Part model, mm, in its own coordinate system. Face numbers are marked on the shaded views. A direction names the side the tool comes from. Give positions to 0.01 mm unless a question says otherwise; leave off trailing zeros. Order: outer loops, then holes, each group sorted by start corner. A loop starts at its lowest first (then second) coordinate and runs counter-clockwise, first axis right, second up. Notation, with made-up numbers: M 11,29.5 L 34,29.5 A18 ccw 34,56.5 Z; hole C 4,79.5 d6. An arc over 180 degrees is marked long. One line per question, with ' | ' between items.
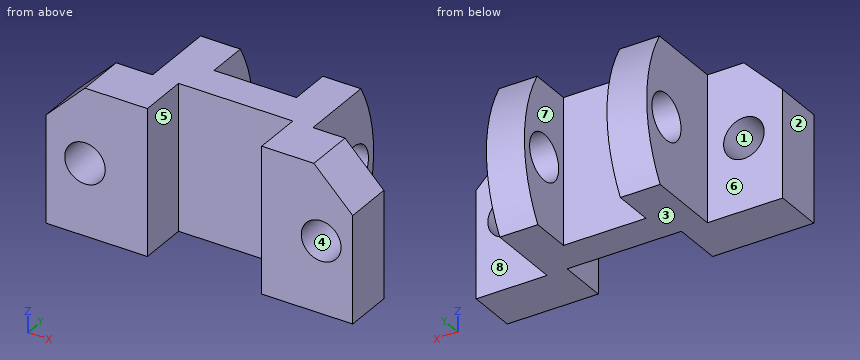
Autodesk Inventor part; units mm, degrees
ref_plane "YZ Plane" through (0, 0, 0) normal (1, 0, 0) x (0, 1, 0)
ref_plane "XZ Plane" through (0, 0, 0) normal (0, 1, 0) x (-1, 0, 0)
ref_plane "XY Plane" through (0, 0, 0) normal (0, 0, 1) x (1, 0, 0)
sketch "스케치1" plane through (0, 0, 0) normal (0, 0, 1) x (1, 0, 0)
  line L0 (31.5724, -15.0322) -> (-31.5724, -15.0322)
  line L1 (-31.5724, -15.0322) -> (-31.5724, 15.0322)
  line L2 (-31.5724, 15.0322) -> (31.5724, 15.0322)
  line L3 (31.5724, 15.0322) -> (31.5724, -15.0322)
  line L4 (31.5724, -15.0322) -> (-31.5724, 15.0322) construction
  line L5 (-31.5724, -15.0322) -> (31.5724, 15.0322) construction
  point P0 (0, 0)
extrude "돌출1" add sketch "스케치1" along normal blind 30
sketch "스케치2" plane through (-31.5724, 15.0322, 0) normal (0, 1, 0) x (1, 0, 0)
  point P0 (31.5724, 0)
sketch "스케치3" plane through (-31.5724, 15.0322, 0) normal (0, 1, 0) x (1, 0, 0)
  line L0 (63.1447, 0) -> (0, 0)
  line L1 (15.5145, 0) -> (15.5145, -30)
  line L2 (0, -30) -> (63.1447, -30)
  line L3 (48.5426, 0) -> (48.5426, -30)
  line L4 (63.1447, -30) -> (0, -30)
  line L5 (15.5145, -30) -> (0, -30)
  line L6 (0, 0) -> (63.1447, 0)
  line L7 (0, -30) -> (0, 0)
  line L8 (0, 0) -> (15.5145, 0)
  line L9 (48.5426, 0) -> (63.1447, 0)
  line L10 (63.1447, 0) -> (63.1447, -30)
  line L11 (63.1447, -30) -> (48.5426, -30)
  line L12 (23.7136, 0) -> (40.7128, 0)
  line L13 (40.7128, 0) -> (40.7128, -30)
  line L14 (40.7128, -30) -> (23.7136, -30)
  line L15 (23.7136, -30) -> (23.7136, 0)
  point P0 (31.5724, 0)
extrude "돌출2" cut sketch "스케치3" against normal blind 20 contours L10 L2 L3 L0 | L1 L2 L7 L0
extrude "돌출3" cut sketch "스케치3" against normal blind 13 contours L13 L2 L15 L0
sketch "스케치4" plane through (0, 0, 30) normal (0, 0, 1) x (1, 0, 0)
  line L0 (-31.5724, -15.0322) -> (31.5724, -15.0322)
  line L1 (-10.7158, -4.9678) -> (12.8298, -4.9678)
  line L2 (12.8298, -4.9678) -> (12.8298, -15.0322)
  line L3 (12.8298, -15.0322) -> (-10.7158, -15.0322)
  line L4 (-10.7158, -15.0322) -> (-10.7158, -4.9678)
  point P0 (0, 0)
extrude "돌출4" cut sketch "스케치4" against normal blind 50
sketch "스케치5" plane through (16.9702, 15.0322, 30) normal (1, 0, 0) x (0, 0, -1)
  circle A0 centre (15.2748, -6.7584) radius 4.7017
  point P0 (30, -15.0322)
extrude "돌출5" cut sketch "스케치5" against normal blind 50
sketch "스케치6" plane through (-31.5724, -4.9678, 0) normal (0, 1, 0) x (1, 0, 0)
  circle A0 centre (56.6423, -14.736) radius 4.1041
  circle A1 centre (7.9978, -14.736) radius 4.1777
  point P0 (31.5724, 0)
extrude "돌출6" cut sketch "스케치6" against normal blind 50
chamfer "모따기1" distance 8 angle 45 2 edges at (-31.5724, -10, 30) (31.5724, -10, 30)
sketch "스케치7" plane through (16.9702, 15.0322, 30) normal (1, 0, 0) x (0, 0, -1)
  point P0 (30, -15.0322)
sketch "스케치8" plane through (16.9702, 15.0322, 30) normal (1, 0, 0) x (0, 0, -1)
  line L0 (30, 0) -> (30, -20)
  line L1 (0, 0) -> (0, -13)
  arc A0 (30, -4.7173) -> (0, -4.4986) centre (14.8208, -29.1901) ccw
  line L2 (0, -4.4986) -> (0, 0)
  line L3 (0, 0) -> (30, 0)
  line L4 (30, 0) -> (30, -4.7173)
  point P0 (30, -15.0322)
extrude "돌출7" cut sketch "스케치8" against normal blind 50
properties part number "240510_3Dsketch07"
1. Slice it at C-C on z = 26. Give the cut face in (x, y), then the cut area to 3 significant figures.
Worked out:
outline: M -27.57,-15.03 L -10.72,-15.03 L -10.72,-4.97 L 12.83,-4.97 L 12.83,-15.03 L 27.57,-15.03 L 27.57,-4.97 L 16.97,-4.97 L 16.97,12.53 L 9.14,12.53 L 9.14,2.03 L -7.86,2.03 L -7.86,12.53 L -16.06,12.53 L -16.06,-4.97 L -27.57,-4.97 Z | area: 717 mm2
2. Slice it at D-D on x = 11.5. Give the cut face in (y, z).
Worked out:
outline: M -4.97,0 L 10.31,0 A28.8 ccw 10.53,30 L -4.97,30 Z; hole C 8.27,14.73 d9.4
3. Slice it at A-A on y = -11.25. Give the cut face in (x, z).
Worked out:
outline: M -31.57,0 L -10.72,0 L -10.72,30 L -23.57,30 L -31.57,22 Z; M 12.83,0 L 31.57,0 L 31.57,22 L 23.57,30 L 12.83,30 Z; hole C -23.57,14.74 d8.36; hole C 25.07,14.74 d8.21
4. Tool access for the marked faces 5, 6, 7 and 8: list every direction of +Z, -Z, +X, -X, +Y, -Y with a clear straight run to the whole face (end or side of a thin tool).
Worked out:
face 5: +Z, -Z, -Y | face 6: +Z, -Z, -X, +Y | face 7: +Z, -Z, +Y | face 8: +Z, -Z, +X, +Y
5. Slice it at B-B on x = -26. Give the cut face in (y, z).
Worked out:
outline: M -15.03,0 L -4.97,0 L -4.97,11.33 L -15.03,11.33 Z; M -15.03,18.14 L -4.97,18.14 L -4.97,27.57 L -15.03,27.57 Z
6. Drop flat-ended pins along their axis: pin 1 (5 mm diameter, centred on x = 25.07, z = 14.74, fed in from +Y); pin 2 (6 mm diameter, centred on y = 0.5, z = 22, fed in from +X); pin 3 (3 mm diameter, centred on x = 2.5, z = 16, fed in from -Y); pin 4 (6 mm diameter, centred on x = -3, z = 25, fed in from +Y). Give the stop position or say it passes through.
Worked out:
pin 1: passes through | pin 2: stops at x = 16.97 | pin 3: stops at y = -4.97 | pin 4: stops at y = 2.03
7. Probe L1, parallel to X at y = -5, z = 6; L2, parallel to X at y = 11, z = 10; L3, parallel to X at y = -6.25, z = 11.5. List the from-to ranges inside material, lowest first. Write a range as from..to.
Worked out:
L1: x = -31.57..-10.72, 12.83..31.57 | L2: x = -16.06..-7.86, 9.14..16.97 | L3: x = -31.57..-26.22, -20.93..-10.72, 12.83..22.55, 27.59..31.57
8. Mould opens along X. For the marked faces 1, 2, 3 and 4 say: released by +X, released by -X, zero draft, split by the parting line, or undercut.
Worked out:
face 1: undercut | face 2: released by -X | face 3: zero draft | face 4: undercut
